The model under review builds one solid part; all positions refer to its coordinate system, in mm. Coordinates: 2 decimals unless noted, no trailing zeros. Write each loop counter-clockwise with the first axis right and the second up, starting at its lowest first coordinate (ties: lowest second). Pieces come first, ordered by that corner, then holes.
Autodesk Inventor part; units mm, degrees
ref_plane "YZ Plane" through (0, 0, 0) normal (1, 0, 0) x (0, 1, 0)
ref_plane "XZ Plane" through (0, 0, 0) normal (0, 1, 0) x (-1, 0, 0)
ref_plane "XY Plane" through (0, 0, 0) normal (0, 0, 1) x (1, 0, 0)
sketch "Sketch1" plane through (0, 0, 0) normal (0, 1, 0) x (-1, 0, 0)
  arc A0 (-1.6679, 36.7922) -> (-1.6679, -36.7922) centre (0, 0) ccw
  arc A1 (157.8679, -44.0244) -> (184, -19.05) centre (159, -19.05) ccw
  arc A2 (184, 19.05) -> (157.8679, 44.0244) centre (159, 19.05) ccw
  line L0 (157.8679, -44.0244) -> (-1.6679, -36.7922)
  line L1 (157.8679, 44.0244) -> (-1.6679, 36.7922)
  line L2 (184, -19.05) -> (184, 19.05)
  line L3 (0, 0) -> (1115.1702, 0)
  dimension "d0" = 50
  dimension "d1" = 159
  dimension "d2" = 38.1
  dimension "d3" = 36.83
extrude "Main" add sketch "Sketch1" along normal blind 3.175
sketch "Sketch2" plane through (0, 3.175, 0) normal (0, 1, 0) x (1, 0, 0)
  circle A0 centre (0, 0) radius 6
  circle A1 centre (-44.4754, 0) radius 20.25
  arc A2 (-184, -19.05) -> (-157.8679, -44.0244) centre (-159, -19.05) ccw
  arc A3 (-157.8679, 44.0244) -> (-184, 19.05) centre (-159, 19.05) ccw
  line L0 (0, 0) -> (-245.2379, 0)
  circle A4 centre (-44.4754, 0) radius 47.5
  line L1 (3.0246, 0) -> (11.0246, 0)
  line L2 (11.0246, 0) -> (11.0246, 5)
  line L3 (11.0246, 5) -> (11.0246, -5)
  line L4 (-91.9754, 0) -> (-99.9754, 0)
  line L5 (-99.9754, 0) -> (-99.9754, 5)
  line L6 (-99.9754, 5) -> (-99.9754, -5)
  circle A5 centre (-99.9754, 5) radius 2.25
  circle A6 centre (-99.9754, -5) radius 2.25
  circle A7 centre (11.0246, 5) radius 2.25
  circle A8 centre (11.0246, -5) radius 2.25
  dimension "d6" = 40.5
  dimension "d40" = 12
  dimension "d41" = 44.4754
  dimension "d77" = 95
  dimension "d78" = 8
  dimension "d79" = 5
  dimension "d80" = 10
  dimension "d81" = 8
  dimension "d82" = 5
  dimension "d83" = 10
  dimension "d84" = 4.5
  dimension "d85" = 4.5
  dimension "d86" = 4.5
  dimension "d87" = 4.5
extrude "Axis Holes" cut sketch "Sketch2" against normal through all contours L1 A4 A0 | A6 | A5 | A0 A4 L1 | A7 | A8 | A4 A0 | L0 A1 | A1 L0
sketch "Sketch5" plane through (0, 3.175, 0) normal (0, 1, 0) x (1, 0, 0)
  line L0 (-133.2, -6.35) -> (-133.2, 29.1375) construction
  line L1 (-184, 19.05) -> (-184, -19.05) construction
  circle A0 centre (-140.2, -6.35) radius 2.75
  circle A1 centre (-150.2, -6.35) radius 2.75
  point P0 (0, 0)
  dimension "d43" = 50.8
  dimension "d44" = 7
  dimension "d45" = 10
  dimension "d46" = 5.5
extrude "Extrusion6" cut sketch "Sketch5" against normal through all
sketch "Sketch9" plane through (0, 3.175, 0) normal (0, 1, 0) x (1, 0, 0)
  circle A0 centre (-44.4754, 0) radius 20.25
  point P0 (0, 0)
  point P1 (-12.3688, -17.5481)
  point P2 (-111.5344, -31)
  point P3 (-111.5344, 31)
  point P4 (22.5836, 0)
  dimension "d73" = 67.059
  dimension "d74" = 67.059
  dimension "d75" = 31
  dimension "d76" = 31
hole "Hole1" at (-111.5344, 3.175, 31) at (-111.5344, 3.175, -31) at (22.5836, 3.175, 0) direction (0, -1, 0) diameter 4.134 end through all countersink diameter 6 countersink angle 90
properties part number "Wrist Side Brase" material "Aluminum 6061"
Item 1: To check wall thickness, follow line 1 along X through (y, z) = (2.95, 7.5); line 2 along Z through (x, y) = (-100, 1.45); line 3 along Z through (x, y) = (-56.5, 0.2). State the ranges of each line that lie inside material, in increasing order.
Solved:
line 1: x = -184 to -152.7, -147.7 to -142.7, -137.7 to -63.29, -25.67 to 36.06
line 2: z = -41.4 to -7.25, -2.75 to 2.75, 7.25 to 41.4
line 3: z = -39.43 to -16.29, 16.29 to 39.43
Item 2: Take a section at A-A, the plane z = 31. Write out the cut boundary in (x, y) (3 decimals), plus the area to 3 significant figures.
Solved:
outline: (-180.959, 0) - (-113.601, 0) - (-113.601, 2.242) - (-114.534, 3.175) - (-180.959, 3.175) - close; (-109.467, 0) - (19.886, 0) - (19.886, 3.175) - (-108.534, 3.175) - (-109.467, 2.242) - close
area: 624 mm2
Item 3: For pin 1 (5 mm diameter, centred on x = -140.2, z = 6.35, fed in from -Y); pin 2 (1.5 mm diameter, centred on x = 4.5, y = 2.5, fed in from -Z); pin 3 (1.5 mm diameter, centred on x = -96.5, y = 2, fed in from +Z), all flat-tipped, find the tip position at first contact; note any pin that passes through.
Solved:
pin 1: passes through
pin 2: stops at z = -36.64
pin 3: stops at z = 41.28
Item 4: Take a section at C-C, the plane y = 1.4. Count the separate pieces of the cut face and the enclosed holes in it, plus the area to 3 significant figures.
Solved:
separate pieces: 1
enclosed holes: 11
area: 15,400 mm2
Item 5: Mouldability with a two-part tool opening along Z and no side actions: class faces 1 (the face through (-97, 3.175, 1)), 2 (the face through (13.103, 1.61, 5.862)), 3 (the face through (-102.223, 1.61, -5.099)), 4 (the face through (36.82, 1.57, -0.79)) as pulls with the +Z half, pulls with the -Z half, needs draft (parallel to the pull), parting line crosses it, or undercut.
Solved:
face 1: needs draft
face 2: undercut
face 3: undercut
face 4: parting line crosses it
Item 6: Take a section at B-B, the plane x = -33.5. Write out the cut boundary in (y, z) (3 decimals), plus the area to 3 significant figures.
Solved:
outline: (0, -38.386) - (3.175, -38.386) - (3.175, -17.018) - (0, -17.018) - close; (0, 17.018) - (3.175, 17.018) - (3.175, 38.386) - (0, 38.386) - close
area: 136 mm2
